Verification items for the finished model (mm, model axes). A direction names the side the tool comes from. Round coordinates to 2 decimals unless told otherwise and drop trailing zeros. Order: outer loops, then holes, each group sorted by start corner. A loop starts at its lowest first (then second) coordinate and runs counter-clockwise, first axis right, second up. Notation, with made-up numbers: (17, 4.25) -> (33, 4.25) arc R22 ccw to (33, 22.25) -> close; hole circle Ø11 at (30, 5.5). An arc over 180 degrees is marked (long way). Put each result on its own line as item: value.
```python
from build123d import *

# Parameters (mm, degrees)
CUT_EXTRUDE1_DEPTH = 1.75


with BuildPart() as part:
    # Sketch2 → Revolve1 (revolve)
    with BuildSketch(Plane(origin=(0, 0, 0), x_dir=(0, 0, -1), z_dir=(1, 0, 0)), mode=Mode.PRIVATE) as revolve1_sk:
        with BuildLine():
            Line((-9.1, 0), (9.1, 0))
            Line((9.1, 0), (9.1, 1.44))
            Line((9.1, 1.44), (8.54, 2))
            Line((8.54, 2), (-6.9, 2))
            Line((-6.9, 2), (-6.9, 3.8))
            Line((-6.9, 3.8), (-7.23, 3.8))
            ThreePointArc((-7.23, 3.8), (-8.306499853, 3.047002626), (-9.1, 2))
            Line((-9.1, 2), (-9.1, 0))
        make_face()
    revolve(revolve1_sk.sketch.rotate(Axis((0, 0, 9.1), (0, 0, -1)), 180), axis=Axis((0, 0, 9.1), (0, 0, -1)))

    # Sketch3 → Cut-Extrude1 (cut)
    with BuildSketch(Plane.XY.offset(9.1)):
        Polygon((0, 1.443375673), (-1.25, 0.721687836), (-1.25, -0.721687836), (0, -1.443375673), (1.25, -0.721687836), (1.25, 0.721687836), align=None)
    extrude(amount=-CUT_EXTRUDE1_DEPTH, mode=Mode.SUBTRACT)

    # Cut-Extrude2 cone 1 section (through the dimple's axis) → Cut-Extrude2 (revolve, cut)
    with BuildSketch(Plane(origin=(0, 0, 9.1), x_dir=(0, -1, 0), z_dir=(1, 0, 0))):
        Polygon((0, 0), (1.443375673, 0), (0, 1.443375673), align=None)
    revolve(axis=Axis((0, 0, 9.1), (0, 0, -1)), mode=Mode.SUBTRACT)


solid = part.part
```
Item 1: Release check for a two-part mould opening along X. For faces 4 (the face through (-1.141, -3.625, 7.067)), 5 (the face through (2, 2, 6.9)), 6 (the face through (-0.63, -1.08, 8.24)) record: pulls with the +X half, pulls with the -X half, needs draft (parallel to the pull), parting line crosses it, or undercut.
Geometry check:
face 4: parting line crosses it
face 5: needs draft
face 6: undercut
Item 2: Sectioned sample at A-A, the plane y = 0. Record the boundary of the cut face in (x, z), then the cut area to 3 significant figures.
Geometry check:
outline: (-3.8, 6.9) -> (-2, 6.9) -> (-2, -8.54) -> (-1.44, -9.1) -> (1.44, -9.1) -> (2, -8.54) -> (2, 6.9) -> (3.8, 6.9) -> (3.8, 7.23) arc R4.23 ccw to (2, 9.1) -> (1.44, 9.1) -> (1.25, 8.91) -> (1.25, 7.35) -> (-1.25, 7.35) -> (-1.25, 8.91) -> (-1.44, 9.1) -> (-2, 9.1) arc R4.23 ccw to (-3.8, 7.23) -> close
area: 73.3 mm2
Item 3: Sectioned sample at B-B, the plane x = -2.5. Record the boundary of the cut face in (y, z), then the cut area to 3 significant figures.
Geometry check:
outline: (-2.86, 6.9) -> (2.86, 6.9) -> (2.86, 7.23) arc R3.41 ccw to (-2.86, 7.23) -> close
area: 8.16 mm2
Item 4: Material ranges on line 1 along Z through (x, y) = (0, -0.5); line 2 along X through (y, z) = (0, -1); line 3 along Z through (x, y) = (1, 1.5), recorded low to high.
Geometry check:
line 1: -9.1 to 7.35
line 2: -2 to 2
line 3: -8.74 to 9.1
Item 5: Depth check by flat-ended pin: pin 1 Ø1.2 at (x, y) = (-0.5, 0.5) entering from +Z; pin 2 Ø4 at (y, z) = (-1.5, -2.5) entering from -X; pin 3 Ø1 at (y, z) = (1.5, -6) entering from -X. Enter the tip coordinate at first touch or a pass-through.
Geometry check:
pin 1: z = 8.96
pin 2: x = -2
pin 3: x = -1.73
Item 6: Sectioned sample at C-C, the plane y = -3. Record the boundary of the cut face in (x, z), then the cut area to 3 significant figures.
Geometry check:
outline: (-2.33, 6.9) -> (2.33, 6.9) -> (2.33, 7.23) arc R2.98 ccw to (-2.33, 7.23) -> close
area: 5.19 mm2
Item 7: Tool access check on faces 1 (the face through (0, 0, -9.1)), 2 (the face through (-1.25, 0, 8)), 3 (the face through (2, 0, -1)). Record the directions out of +Z, -Z, +X, -X, +Y, -Y that give a thin tool (end or side, any length) a straight path to the whole face; none if there is none.
Geometry check:
face 1: -Z, +X, -X, +Y, -Y
face 2: +Z
face 3: -Z
